Autodesk Inventor part; units mm, degrees
ref_plane "Arbeitsebene1" through (-18.125, 0, 0) normal (0, -1, 0) x (1, 0, 0)
ref_plane "YZ Plane" through (0, 0, 0) normal (1, 0, 0) x (0, 1, 0)
ref_plane "XZ Plane" through (0, 0, 0) normal (0, 1, 0) x (-1, 0, 0)
sketch "Skizze1" plane through (0, 0, 0) normal (0, 0, 1) x (1, 0, 0)
  circle A0 centre (0, 18.125) radius 1.4
  circle A1 centre (-18.125, 0) radius 1.4
  circle A2 centre (0, -18.125) radius 1.4
  circle A3 centre (18.125, 0) radius 1.4
  circle A4 centre (0, 0) radius 11.25
  circle A5 centre (0, 0) radius 25
  circle A6 centre (0, 0) radius 24.5
  line L0 (-18.125, 0) -> (18.125, 0)
  circle A7 centre (0, 0) radius 13
  point P0 (0, 0)
  dimension "d0" = 49
  dimension "d19" = 26
extrude "Extrusion1" add sketch "Skizze1" along normal blind 4 contours A7 L0 A4 | L0 A4 A7 | A6
sketch "Skizze2" plane through (0, 0, 4) normal (0, 0, 1) x (1, 0, 0)
  circle A0 centre (0, 0) radius 11.25
  circle A1 centre (18.125, 0) radius 1.4
  circle A2 centre (0, -18.125) radius 1.4
  circle A3 centre (-18.125, 0) radius 1.4
  circle A4 centre (0, 18.125) radius 1.4
  circle A5 centre (0, 0) radius 24.5
ref_plane "Arbeitsebene1" through (-18.125, 0, 0) normal (0, -1, 0) x (1, 0, 0)
sketch "Skizze3" plane through (-18.125, 0, 0) normal (0, -1, 0) x (1, 0, 0)
  line L0 (34.85, 4) -> (34.85, 0)
  line L1 (34.85, 0) -> (29.375, 0)
  line L2 (29.375, 0) -> (29.375, 4)
  line L3 (29.375, 4) -> (34.85, 4)
  line L4 (1.4, 0) -> (1.4, 4)
  line L5 (1.4, 4) -> (6.875, 4)
  line L6 (6.875, 4) -> (6.875, 0)
  line L7 (6.875, 0) -> (1.4, 0)
  line L8 (-6.375, 0) -> (-6.375, 4)
  line L9 (-6.375, 4) -> (-1.4, 4)
  line L10 (-1.4, 4) -> (-1.4, 0)
  line L11 (-1.4, 0) -> (-6.375, 0)
  line L12 (42.625, 4) -> (42.625, 0)
  line L13 (42.625, 0) -> (37.65, 0)
  line L14 (37.65, 0) -> (37.65, 4)
  line L15 (37.65, 4) -> (42.625, 4)
  arc A0 (18.125, 6) -> (-6.375, 4) centre (18.125, -145.0625) ccw
  line L16 (18.125, 6) -> (18.125, 4)
  line L17 (18.125, 4) -> (-6.375, 4)
  line L18 (18.125, 18.126) -> (18.125, -80.6859)
  point P0 (18.125, 0)
  dimension "d4" = 2
revolve "Umdrehung1" add sketch "Skizze3" angle 360 about axis through (0, 0, 6) along (0, 0, -1) contours L17 L9 A0 L16 L5
sketch "Skizze4" plane through (0, 0, 0) normal (0, 0, -1) x (-1, 0, 0)
  circle A0 centre (-18.125, 0) radius 1.4
  circle A1 centre (0, -18.125) radius 1.4
  circle A2 centre (18.125, 0) radius 1.4
  circle A3 centre (0, 18.125) radius 1.4
hole "Bohrung1" at (18.125, 0, 0) at (0, -18.125, 0) at (-18.125, 0, 0) at (0, 18.125, 0) direction (0, 0, 1) diameter 3.3 end through all
chamfer "Fase1" distance 2 angle 45 6 edges at (-16.961, 1.1694, 5.0403) (-19.2889, 1.1696, 4.7589) (-18.1249, -1.65, 4.8996) (0, 16.475, 5.0989) (18.1248, -1.65, 4.8997) (0, -19.775, 4.7001)
sketch "Skizze5" plane through (0, 0, 0) normal (0, 0, -1) x (-1, 0, 0)
  circle A0 centre (0, 0) radius 11.25
  circle A1 centre (0, 0) radius 13.5
  dimension "d20" = 27
extrude "Extrusion2" cut sketch "Skizze5" against normal up to surface (4 mm away)
properties part number "Abdeckung" material "ABS-Kunststoff - Orange"
Source: CAD feature listing. Evaluate the final solid. Frame: model axes, mm. A direction names the side the tool comes from. Coordinates: 2 decimals unless noted, no trailing zeros. Loops run counter-clockwise (first coordinate to the right, second up) from the corner with the lowest first, then second, coordinate; pieces in that order, holes last. Notation, with made-up numbers: (46.5, 85) - (71.5, 85) arc R4 ccw to (71.5, 89) - close; hole circle Ø10 at (19, 80.5). An arc over 180 degrees is marked (long way). Return JSON: item names as keys, results as strings.
Q1. Section D-D, the plane x = 0. Give the number of separate pieces and of enclosed holes in the cut face, plus the area to 3 significant figures.
Results:
{"separate pieces": "3", "enclosed holes": "0", "area": "113 mm2"}
Q2. Contact query for flat-ended pins moving along their axis: P1, Ø1, axis at x = 14, y = 6.5, coming from the +Z side; P2, Ø13.5, axis at x = -1.5, y = -2, coming from the -Z side; P3, Ø1.5, axis at x = 7.5, z = 4, coming from the -Y side. Output: stop coordinate, or through.
Results:
{"P1": "z = 5.26", "P2": "z = 4", "P3": "y = -23.55"}
Q3. Mould query, pull axis Y, two halves, no side actions, for faces 3 (the cylindrical face through (-0.496, -16.551, 1.571)), 4 (the cylindrical face through (13.17, -20.66, 1.97)), 5 (the flat face through (11, -11, 0)). Classes: released by +Y, released by -Y, zero draft, split by the parting line, or undercut.
Results:
{"face 3": "undercut", "face 4": "split by the parting line", "face 5": "zero draft"}
Q4. Access query for faces 1 (the flat face through (0, 0, 4)), 2 (the cylindrical face through (-0.073, 16.477, 1.571)). Directions: +Z, -Z, +X, -X, +Y, -Y. A direction counts if a zero-diameter tool reaches every point of the face in a straight line with its end or side. Return the directions, or none.
Results:
{"face 1": "-Z", "face 2": "+Z, -Z"}
Q5. Material intervals for line 1 along Y through (x, z) = (0, 2) (3 decimals); line 2 along Y through (x, z) = (1, 3.5); line 3 along Y through (x, z) = (5, 2), sorted ascending.
Results:
{"line 1": "-24.5 to -19.775, -16.475 to -13.5, 13.5 to 16.475, 19.775 to 24.5", "line 2": "-24.48 to -20.46, -16.34 to -13.46, 13.46 to 16.34, 20.46 to 24.48", "line 3": "-23.98 to -12.54, 12.54 to 23.98"}
Q6. Section A-A, the plane y = -8. Return loops of the section in (x, z).
Results:
{"outline": "(-23.16, 0) - (-10.87, 0) - (-10.87, 4) - (10.87, 4) - (10.87, 0) - (23.16, 0) - (23.16, 4) arc R150.85 ccw to (-23.16, 4) - close"}
Q7. Section B-B, the plane z = 1.5. Return loops of the section in (x, y) (3 decimals), plus the area to 3 significant figures.
Results:
{"outline": "circle Ø49 at (0, 0); hole circle Ø3.3 at (-18.125, 0); hole circle Ø27 at (0, 0); hole circle Ø3.3 at (0, -18.125); hole circle Ø3.3 at (0, 18.125); hole circle Ø3.3 at (18.125, 0)", "area": "1,280 mm2"}
Q8. Section C-C, the plane x = 6.5. Return loops of the section in (y, z), plus the area to 3 significant figures.
Results:
{"outline": "(-23.62, 0) - (-11.83, 0) - (-11.83, 4) - (11.83, 4) - (11.83, 0) - (23.62, 0) - (23.62, 4) arc R150.92 ccw to (-23.62, 4) - close", "area": "153 mm2"}
